Can you work these out from the model? Positions are in its coordinate system, mm. Round coordinates to 2 decimals unless told otherwise and drop trailing zeros. Write each loop counter-clockwise with the first axis right and the second up, starting at its lowest first coordinate (ties: lowest second). Pieces come first, ordered by that corner, then holes. Notation, with made-up numbers: M 78.5,6.25 L 109.5,6.25 A24 ccw 109.5,42.25 Z; hole C 83,6.25 d8. An arc over 180 degrees is marked long. Answer as a JSON object with one key per item and string values. Group by question number.
1) Suppose I cut it at C-C, the plane y = 1.1. Write out the boundary of the cut face in (x, z), and give its area (3 significant figures).
2) Suppose I cut it at B-B, the plane z = 0. Write out the boundary of the cut face in (x, y) (3 decimals), and give its area (3 significant figures).
3) I'm going to push flat-ended pins straight in: pin 1 Ø10 at (x, z) = (17, -27) entering from -Y; pin 2 Ø2 at (x, z) = (40, 0) entering from -Y; pin 3 Ø1 at (x, y) = (25.5, 0.5) entering from +Z; pin 4 Ø1.5 at (y, z) = (2, 18) entering from -X. Where does each tip first touch, or does it pass through?
4) Please list where these lines run through material, in increasing order: L1, parallel to Z at x = -1, y = 1.55; L2, parallel to Z at x = -6, y = 0.1; L3, parallel to X at y = 1.5, z = 7. Write a range as [from, to].
5) Suppose I cut it at D-D, the plane z = -16. Write out the boundary of the cut face in (x, y), and give its area (3 significant figures).
6) Suppose I cut it at A-A, the plane x = 0. Write out the boundary of the cut face in (y, z).
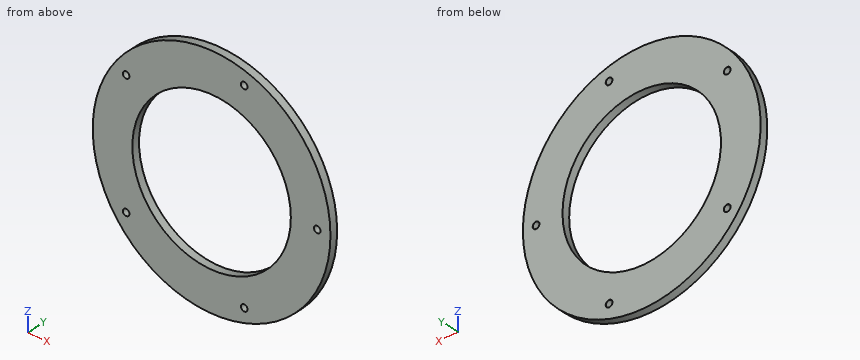
from build123d import *

# Parameters (mm, degrees)
SKETCH_1_R                   = 45
EXTRUDE_1_DEPTH              = 3
SKETCH_5_R                   = 30
CUT_EXTRUDE_1_DEPTH          = 1
CUT_EXTRUDE_1_DEPTH_BACK     = 4
HOLE_WIZARD_M3_2_D           = 2.5
HOLE_WIZARD_M3_2_CSINK_D     = 2.55
HOLE_WIZARD_M3_2_CSINK_ANGLE = 90


with BuildPart() as part:
    # 草图1 → 凸台-拉伸1 (new body)
    with BuildSketch(Plane(origin=(0, 0, 0), x_dir=(1, 0, 0), z_dir=(0, 1, 0))):
        Circle(SKETCH_1_R)
    extrude(amount=EXTRUDE_1_DEPTH)

    # 草图5 → 切除-拉伸1 (cut, two sides)
    with BuildSketch(Plane(origin=(0, 3, 0), x_dir=(1, 0, 0), z_dir=(0, 1, 0))) as cut_extrude_1_sk:
        Circle(SKETCH_5_R)
    extrude(amount=CUT_EXTRUDE_1_DEPTH, mode=Mode.SUBTRACT)
    extrude(cut_extrude_1_sk.sketch, amount=-CUT_EXTRUDE_1_DEPTH_BACK, mode=Mode.SUBTRACT)

    # M3 螺纹孔的螺纹孔钻头2 (through all)
    with Locations(Plane(origin=(0, 3, 0), x_dir=(1, 0, 0), z_dir=(0, 1, 0))):
        with Locations((0, 0), (40, 0), (12.360679775, -38.042260652), (-32.360679775, -23.511410092), (-32.360679775, 23.511410092), (12.360679775, 38.042260652)):
            CounterSinkHole(HOLE_WIZARD_M3_2_D / 2, HOLE_WIZARD_M3_2_CSINK_D / 2, counter_sink_angle=HOLE_WIZARD_M3_2_CSINK_ANGLE)


solid = part.part
Results:
{
 "1": {"outline": "C 0,0 d90; hole C -32.36,-23.51 d2.5; hole C -32.36,23.51 d2.5; hole C 0,0 d60; hole C 12.36,-38.04 d2.5; hole C 12.36,38.04 d2.5; hole C 40,0 d2.5", "area": "3,510 mm^2"},
 "2": {"outline": "M -45,0 L -30,0 L -30,3 L -45,3 Z; M 30,0 L 38.75,0 L 38.75,2.975 L 38.725,3 L 30,3 Z; M 41.25,0 L 45,0 L 45,3 L 41.275,3 L 41.25,2.975 Z", "area": "82.5 mm^2"},
 "3": {"pin 1": "y = 0", "pin 2": "through", "pin 3": "z = 37.42", "pin 4": "x = -41.56"},
 "4": {"L1": "[-44.99, -29.98], [29.98, 44.99]", "L2": "[-44.6, -29.39], [29.39, 44.6]", "L3": "[-44.45, -29.17], [29.17, 44.45]"},
 "5": {"outline": "M -42.06,0 L -25.38,0 L -25.38,3 L -42.06,3 Z; M 25.38,0 L 42.06,0 L 42.06,3 L 25.38,3 Z", "area": "100 mm^2"},
 "6": {"outline": "M 0,-45 L 3,-45 L 3,-30 L 0,-30 Z; M 0,30 L 3,30 L 3,45 L 0,45 Z"}
}
